For this review, take the finished solid that the model builds, in its own axes (mm). A direction names the side the tool comes from. Round coordinates to 2 decimals unless told otherwise and drop trailing zeros. Loops run counter-clockwise (first coordinate to the right, second up) from the corner with the lowest first, then second, coordinate; pieces in that order, holes last.
1. Consider section B-B on y = 51. State the section outline as (x, z) points.
2. Tool access review of faces 1 (the flat face through (-49, 128, -85)), 2 (the cylindrical face through (-71.34, 0.14, -7)), 3 (the cylindrical face through (-44.28, -43.61, 1.58)), 4 (the cylindrical face through (0.279, 87.297, 1.578)): name each direction out of +Z, -Z, +X, -X, +Y, -Y from which nothing blocks a thin tool from reaching the whole face with its end or side.
3. Consider section A-A on z = -3.5. State the section outline as (x, y) points.
4. Draft analysis for pull direction X (two halves, no side actions). For faces 5 (the cylindrical face through (-57.095, 2.513, 3.94)), 6 (the flat face through (-60, -25, 0)), 7 (the cylindrical face through (0.708, -77.786, -6.995)), state which applies: released by +X, released by -X, zero draft, split by the parting line, or undercut.
5. Consider section D-D on z = -124. State the section outline as (x, y) points.
6. To check wall thickness, follow line 1 along X through (y, z) = (0, -3); line 2 along Z through (x, y) = (-10, -60.5); line 3 along X through (y, z) = (74.6, -5). State the ranges of each line that lie inside material, in increasing order.
7. Clearance check with flat-ended pins moving along their axes: pin 1 Ø2.5 at (y, z) = (-69.5, 2.5) entering from +X; pin 2 Ø3 at (y, z) = (6.5, 0) entering from -X; pin 3 Ø1.6 at (y, z) = (70, 2) entering from -X. State where each tip first meets the part, or that it passes through.
8. Consider section C-C on x = -34.5. State the section outline as (y, z) points (3 decimals).
from build123d import *

# Parameters (mm, degrees)
SKETCH1_R                    = 130
BOSS_EXTRUDE1_DEPTH          = 172
BOSS_EXTRUDE2_DEPTH          = 3.2
SKETCH3_R                    = 57.15
BOSS_EXTRUDE3_DEPTH          = 1.5
F_5_16_18_TAPPED_HOLE1_D     = 6.5278
F_5_16_18_TAPPED_HOLE1_DEPTH = 20.1091
F_5_16_18_TAPPED_HOLE1_TIP   = 1.961148974
SKETCH6_W                    = 98
SKETCH6_H                    = 47.7
BOSS_EXTRUDE4_DEPTH          = 172
BOSS_EXTRUDE5_DEPTH          = 42.6


with BuildPart() as part:
    # Sketch1 → Boss-Extrude1 (new body)
    with BuildSketch(Plane.XY):
        Circle(SKETCH1_R)
    extrude(amount=-BOSS_EXTRUDE1_DEPTH)

    # Sketch2 → Boss-Extrude2 (add)
    with BuildSketch(Plane.XY):
        with BuildLine():
            Line((-63.229996837, 12.7), (-74.6, 12.7))
            ThreePointArc((-74.6, 12.7), (-87.3, 0), (-74.6, -12.7))
            Line((-74.6, -12.7), (-63.229996837, -12.7))
            ThreePointArc((-63.229996837, -12.7), (-61.381868207, -13.336862135), (-60.318408341, -14.977052955))
            ThreePointArc((-60.318408341, -14.977052955), (-43.946686451, -43.946686451), (-14.977052955, -60.318408341))
            ThreePointArc((-14.977052955, -60.318408341), (-13.336862135, -61.381868207), (-12.7, -63.229996837))
            Line((-12.7, -63.229996837), (-12.7, -74.6))
            ThreePointArc((-12.7, -74.6), (0, -87.3), (12.7, -74.6))
            Line((12.7, -74.6), (12.7, -63.229996837))
            ThreePointArc((12.7, -63.229996837), (13.336862135, -61.381868207), (14.977052955, -60.318408341))
            ThreePointArc((14.977052955, -60.318408341), (43.946686451, -43.946686451), (60.318408341, -14.977052955))
            ThreePointArc((60.318408341, -14.977052955), (61.381868207, -13.336862135), (63.229996837, -12.7))
            Line((63.229996837, -12.7), (74.6, -12.7))
            ThreePointArc((74.6, -12.7), (87.3, 0), (74.6, 12.7))
            Line((74.6, 12.7), (63.229996837, 12.7))
            ThreePointArc((63.229996837, 12.7), (61.381868207, 13.336862135), (60.318408341, 14.977052955))
            ThreePointArc((60.318408341, 14.977052955), (43.946686451, 43.946686451), (14.977052955, 60.318408341))
            ThreePointArc((14.977052955, 60.318408341), (13.336862135, 61.381868207), (12.7, 63.229996837))
            Line((12.7, 63.229996837), (12.7, 74.6))
            ThreePointArc((12.7, 74.6), (0, 87.3), (-12.7, 74.6))
            Line((-12.7, 74.6), (-12.7, 63.229996837))
            ThreePointArc((-12.7, 63.229996837), (-13.336862135, 61.381868207), (-14.977052955, 60.318408341))
            ThreePointArc((-14.977052955, 60.318408341), (-43.946686451, 43.946686451), (-60.318408341, 14.977052955))
            ThreePointArc((-60.318408341, 14.977052955), (-61.381868207, 13.336862135), (-63.229996837, 12.7))
        make_face()
    extrude(amount=BOSS_EXTRUDE2_DEPTH)

    # Sketch3 → Boss-Extrude3 (add)
    with BuildSketch(Plane.XY.offset(3.2)):
        Circle(SKETCH3_R)
    extrude(amount=BOSS_EXTRUDE3_DEPTH)

    # 5/16-18 Tapped Hole1
    with Locations(Plane.XY.offset(3.2)):
        with Locations((-74.6, 0), (0, 74.6), (74.6, 0), (0, -74.6)):
            Hole(F_5_16_18_TAPPED_HOLE1_D / 2, depth=F_5_16_18_TAPPED_HOLE1_DEPTH)
            with Locations((0, 0, -(F_5_16_18_TAPPED_HOLE1_DEPTH + F_5_16_18_TAPPED_HOLE1_TIP / 2))):  # 118° drill point
                Cone(0, F_5_16_18_TAPPED_HOLE1_D / 2, F_5_16_18_TAPPED_HOLE1_TIP, mode=Mode.SUBTRACT)

    # Sketch6 → Boss-Extrude4 (add)
    with BuildSketch(Plane.XY):
        with Locations((0, 111.15)):
            Rectangle(SKETCH6_W, SKETCH6_H)
    extrude(amount=-BOSS_EXTRUDE4_DEPTH)

    # Sketch7 → Boss-Extrude5 (add)
    with BuildSketch(Plane.XY.offset(4.7)):
        with BuildLine():
            Line((-2.39, 10.855004606), (-2.39, 8.205004606))
            Line((-2.39, 8.205004606), (2.39, 8.205004606))
            Line((2.39, 8.205004606), (2.39, 10.855004606))
            ThreePointArc((2.39, 10.855004606), (0, -11.115), (-2.39, 10.855004606))
        make_face()
    extrude(amount=BOSS_EXTRUDE5_DEPTH)


solid = part.part
Resolved:
1. outline: (-119.58, -172) - (119.58, -172) - (119.58, 0) - (35.52, 0) - (35.52, 3.2) - (25.79, 3.2) - (25.79, 4.7) - (-25.79, 4.7) - (-25.79, 3.2) - (-35.52, 3.2) - (-35.52, 0) - (-119.58, 0) - close
2. face 1: +Z, -Z, -X, +Y
2. face 2: +Z
2. face 3: +Z, -X, -Y
2. face 4: +Z, +Y
3. outline: (-49, 120.41) arc R130 ccw (long way) to (49, 120.41) - (49, 135) - (-49, 135) - close; hole circle Ø6.53 at (-74.6, 0); hole circle Ø6.53 at (0, -74.6); hole circle Ø6.53 at (0, 74.6); hole circle Ø6.53 at (74.6, 0)
4. face 5: split by the parting line
4. face 6: zero draft
4. face 7: undercut
5. outline: (-49, 120.41) arc R130 ccw (long way) to (49, 120.41) - (49, 135) - (-49, 135) - close
6. line 1: x = -130 to -77.86, -71.34 to 71.34, 77.86 to 130
6. line 2: z = -172 to 3.2
6. line 3: x = -106.47 to -3.26, 3.26 to 106.47
7. pin 1: stops at x = 12.7
7. pin 2: stops at x = -129.9
7. pin 3: stops at x = -12.7
8. outline: (-125.339, -172) - (135, -172) - (135, 0) - (51.695, 0) - (51.695, 3.2) - (45.562, 3.2) - (45.562, 4.7) - (-45.562, 4.7) - (-45.562, 3.2) - (-51.695, 3.2) - (-51.695, 0) - (-125.339, 0) - close
